Verification items for the finished model (mm, model axes). A direction names the side the tool comes from. Round coordinates to 2 decimals unless told otherwise and drop trailing zeros. Write each loop counter-clockwise with the first axis right and the second up, starting at its lowest first coordinate (ties: lowest second). Pieces come first, ordered by that corner, then holes. Notation, with made-up numbers: M 86.5,51 L 92.5,51 A17 ccw 92.5,66 Z; hole C -6.75,-23 d4. An arc over 180 degrees is marked long. Answer in a Markdown table with one row per item. Add a question column.
1. Set-up check for faces 1 (the cylindrical face through (0, 1.5, -12.9)), 2 (the flat face through (0, 2, 15)), 3 (the cylindrical face through (-0.1, 3.5, -2.9)): record each of +Z, -Z, +X, -X, +Y, -Y from which the full face is reachable in a straight line by a thin tool's end or side.
2. Sectioned sample at C-C on y = 5.5. Record the cut outline in (x, z).
3. Draft check along Z on faces 4 (the flat face through (0, 3, 0)), 5 (the conical face through (0.06, 2.79, -22.33)), 6 (the cylindrical face through (0.05, 2.4, 7.6)). Enter one of: pulls with the +Z half, pulls with the -Z half, needs draft (parallel to the pull), parting line crosses it, or undercut.
4. Sectioned sample at B-B on z = 3. Record the cut outline in (x, y).
5. Go/stop test with flat-tipped pins: pin 1 Ø4 at (x, z) = (-3.5, -46.5) entering from +Y; pin 2 Ø1.5 at (x, z) = (3, -20) entering from +Y; pin 3 Ø2 at (y, z) = (3.5, -47) entering from -X. Record where each tip stops, or that it passes through.
6. Material ranges on probe 1 along Z at (x, y) = (-6, 6); probe 2 along Z at (x, y) = (6.5, 2); probe 3 along X at (y, z) = (1, -24), recorded low to high.
7. Sectioned sample at A-A on x = 0. Record the cut outline in (y, z), plus the area to 3 significant figures.
8. Sectioned sample at D-D on z = -53.5. Record the cut outline in (x, y).
Autodesk Inventor part; units mm, degrees
ref_plane "YZ Plane" through (0, 0, 0) normal (1, 0, 0) x (0, 1, 0)
ref_plane "XZ Plane" through (0, 0, 0) normal (0, 1, 0) x (-1, 0, 0)
ref_plane "XY Plane" through (0, 0, 0) normal (0, 0, 1) x (1, 0, 0)
sketch "Sketch1" plane through (0, 0, 0) normal (0, 1, 0) x (-1, 0, 0)
  line L0 (0, 0) -> (-1.5, 0)
  line L1 (-1.5, 0) -> (-3.5, 0)
  line L2 (0, 0) -> (0, -40.75)
  line L3 (0, -40.75) -> (0, -50.75)
  circle A0 centre (0, -50.75) radius 10
  line L4 (-1.5, -40.8631) -> (0, -40.8631)
  line L5 (0, -40.8631) -> (0, -40.75)
  line L6 (-1.5, -40.8631) -> (-1.5, 0)
  line L7 (0, -40.75) -> (-1.5, -40.75)
  line L8 (-1.5, -40.75) -> (-2, -40.75)
  line L9 (0, -50.75) -> (0, -60.75)
  circle A1 centre (0, -50.75) radius 9.2
  line L10 (-1.5, 0) -> (-1.5, 15)
  line L11 (-3.5, 0) -> (-3.5, 15)
  line L12 (-3.5, 15) -> (-1.5, 15)
  arc A2 (-3.3801, -41.3386) -> (-2.0575, -39.3831) centre (-4.0561, -39.4563) ccw
  line L13 (-1.5, -40.8631) -> (-1.5, -41.6731)
  line L14 (0, 0) -> (-2.4, 0)
  line L15 (-2.4, 0) -> (-2.4, 15)
  line L16 (0, 0) -> (-1.5, 0)
  line L17 (-1.5, 0) -> (-1.5, 15)
  line L18 (-2.4, 15) -> (0, 15)
  line L19 (0, 15) -> (0, 0)
  line L20 (-1.5, 0) -> (-1.5, 0)
  line L21 (-1.5, 0) -> (-1.5, -2)
  line L22 (-1.5, -2) -> (-1.5, -2)
  line L23 (-3.5, 0) -> (-3.5, -5.75)
  line L24 (-3.5, -5.75) -> (-2.0575, -39.3831)
  point P0 (0, -59.95)
  point P1 (0, -41.55)
  dimension "d7" = 18.4
  dimension "d1" = 2
  dimension "d2" = 40.75
  dimension "d4" = 10
  dimension "d9" = 15
  dimension "d16" = 1.5
  dimension "d19" = 2
  dimension "d20" = 2.4
  dimension "d21" = 15
  dimension "d22" = 1.5
  dimension "d23" = 2
  dimension "d24" = 3.5
  dimension "d25" = 5.75
revolve "Revolution1" add sketch "Sketch1" angle 180 about axis through (0, 0, 0) along (0, 0, 1) contours L6 A0 A2 L24 L23 L1 | L1 L15 L12 L10 | L13 A1 L9 A0
sketch "Sketch2" plane through (3.7, 0, 0) normal (0, 0, 1) x (1, 0, 0)
  circle A0 centre (-3.7, 0) radius 3.7
  circle A1 centre (-3.7, 0) radius 2.2
  line L0 (-0.2, 0) -> (-1.6425, 0)
  line L1 (0, 0) -> (-7.4, 0)
  point P0 (-1.7, 0)
  point P1 (-5.9, 0)
  point P2 (-1.5, 0)
  dimension "d13" = 4.4
  dimension "d14" = 7.4
extrude "Rod Stopper" [suppressed]
equation "\"d23\" = d1"
properties part number "markerWithRodEnd_3DPrint"
Geometry check:
| question | item | result |
|---|---|---|
| 1 | face 1 | +Z, -Y |
| 1 | face 2 | +Z, +X, -X, +Y, -Y |
| 1 | face 3 | +Z, +Y |
| 2 | outline | C 0,-50.75 d16.7; hole C 0,-50.75 d14.75 |
| 3 | face 4 | pulls with the +Z half |
| 3 | face 5 | undercut |
| 3 | face 6 | needs draft |
| 4 | outline | M -2.4,0 L -1.5,0 A1.5 cw 1.5,0 L 2.4,0 A2.4 ccw Z |
| 5 | pin 1 | stops at y = 9.37 |
| 5 | pin 2 | stops at y = 1.81 |
| 5 | pin 3 | stops at x = -9.11 |
| 6 | probe 1 | z = -56.04 to -54.31, -47.19 to -45.46 |
| 6 | probe 2 | z = -58.08 to -56.95, -44.55 to -43.42 |
| 6 | probe 3 | x = -2.53 to -1.12, 1.12 to 2.53 |
| 7 | outline | M 0,-60.75 A10 ccw 3.38,-41.34 A2 cw 2.06,-39.38 L 3.5,-5.75 L 3.5,0 L 2.4,0 L 2.4,15 L 1.5,15 L 1.5,-41.67 A9.2 cw 0,-59.95 Z |
| 7 | area | 92.2 mm2 |
| 8 | outline | M -9.61,0 L -8.78,0 A8.78 cw 8.78,0 L 9.61,0 A9.61 ccw Z |
